Build history of the part. All positions in model axes, mm. Give positions to 0.01 mm unless a question says otherwise; leave off trailing zeros. Order: outer loops, then holes, each group sorted by start corner. A loop starts at its lowest first (then second) coordinate and runs counter-clockwise, first axis right, second up. Notation, with made-up numbers: (-6.5, 47) -> (14.5, 47) arc R17 ccw to (14.5, 62) -> close; hole circle Ø6 at (84.5, 16.5). An arc over 180 degrees is marked (long way). One line per question, with ' | ' between items. Start each with the question number.
(1) Drill centre lines: L1, parallel to X at y = -3, z = 0.5; L2, parallel to X at y = -2.45, z = -3; L3, parallel to Z at x = -3, y = -2. Where is each one in solid material? Low to high. Write a range as from..to.
(2) Cut at A-A (x = -0.5). Give the cut face in (y, z) (3 decimals).
(3) Pin check, flat tip, straight feed: pin 1 Ø1 at (x, y) = (26.5, -2) entering from +Z. Stop position of the tip, or through.
(4) Pull direction Y, two halves, no side cores. Call faces 1 (the face through (31.69, -1.57, -1.94)), 2 (the face through (9, 0, 1)), 3 (the face through (9, -3.175, 1)): +Y half, -Y half, draft (parallel to the pull), parting line (faces both ways), or undercut.
from build123d import *

# Parameters (mm, degrees)
F1_DEPTH = 3.175
F2_R     = 5


# Not quite as in the source:
# - a length typed as a fraction of an inch, garbled in the dataset ("3 / 203.2 mm" for 3/8 in), is restored


with BuildPart() as f1:
    # F0 (on Front) → F1 (new body)
    with BuildSketch(Plane.XZ):
        with BuildLine():
            ThreePointArc((5, 0), (4.7976890268, 1.4078991449), (4.2071279991, 2.7018649113))
            ThreePointArc((4.2071279991, 2.7018649113), (0.0116152193, 4.9999865086), (-4.1945295238, 2.7213823829))
            ThreePointArc((-4.1945295238, 2.7213823829), (-4.3935698421, -2.3867433969), (0, -5))
            add(Edge.make_bspline(
                [(0, -5), (0.5720738613, -4.9218364583), (1.1062852924, -4.8328629446), (1.6070336906, -4.7347061912)],
                knots=[0, 0, 0, 0, 0.0353074902, 0.0353074902, 0.0353074902, 0.0353074902], degree=3))
            ThreePointArc((1.6070336906, -4.7347061912), (3.070488906, -3.9461497536), (4.1945295238, -2.7213823829))
            ThreePointArc((4.1945295238, -2.7213823829), (4.7944054699, -1.4190405881), (5, 0))
        make_face()
        with BuildLine():
            ThreePointArc((1.3244951977, 0.8751392582), (1.5203276582, 0.4569026831), (1.5875, 0))
            ThreePointArc((1.5875, 0), (-1.5203276582, -0.4569026831), (1.3244951977, 0.8751392582))
        make_face(mode=Mode.SUBTRACT)
        with BuildLine():
            add(Edge.make_bspline(
                [(4.2071279991, 2.7018649113), (8.5330066632, 5.3268453963), (13.9608292527, 6.9611647512), (24.1781340673, 4.7387528577), (32.5091555715, 0)],
                knots=[0.1019845344, 0.1019845344, 0.1019845344, 0.1019845344, 0.46554979, 1, 1, 1, 1], degree=3))
            ThreePointArc((4.2071279991, 2.7018649113), (4.7976890268, 1.4078991449), (5, 0))
            ThreePointArc((5, 0), (4.7944054699, -1.4190405881), (4.1945295238, -2.7213823829))
            ThreePointArc((4.1945295238, -2.7213823829), (3.070488906, -3.9461497536), (1.6070336906, -4.7347061912))
            add(Edge.make_bspline(
                [(1.6070336906, -4.7347061912), (7.7069500406, -3.5389999501), (10.2510979188, 2.1993831398), (27.8217853485, 0), (30.8888312429, -3.8289688528)],
                knots=[0.0353074902, 0.0353074902, 0.0353074902, 0.0353074902, 0.4654091895, 1, 1, 1, 1], degree=3))
            Line((30.8888312429, -3.8289688528), (32.5091555715, 0))
        make_face()
        with BuildLine():
            add(Edge.make_bspline(
                [(0, -5), (0.5720738613, -4.9218364583), (1.1062852924, -4.8328629446), (1.6070336906, -4.7347061912)],
                knots=[0, 0, 0, 0, 0.0353074902, 0.0353074902, 0.0353074902, 0.0353074902], degree=3))
            ThreePointArc((0, -5), (0.814392118, -4.9332307343), (1.6070336906, -4.7347061912))
        make_face()
    extrude(amount=F1_DEPTH)

    # F2
    f2_edges = [f1.edges().sort_by_distance(p)[0] for p in [
        (4.207128, -1.5875, 2.701865),
    ]]
    fillet(f2_edges, radius=F2_R)


solid = f1.part
Result set:
1) L1: x = -4.97..-1.51, 1.51..31.62 | L2: x = -4..6.74, 30.08..31.24 | L3: z = -4..4
2) outline: (-3.175, -4.975) -> (0, -4.975) -> (0, -1.507) -> (-3.175, -1.507) -> close; (-3.175, 1.507) -> (0, 1.507) -> (0, 4.975) -> (-3.175, 4.975) -> close
3) pin 1: stops at z = 3.23
4) face 1: draft | face 2: +Y half | face 3: -Y half
